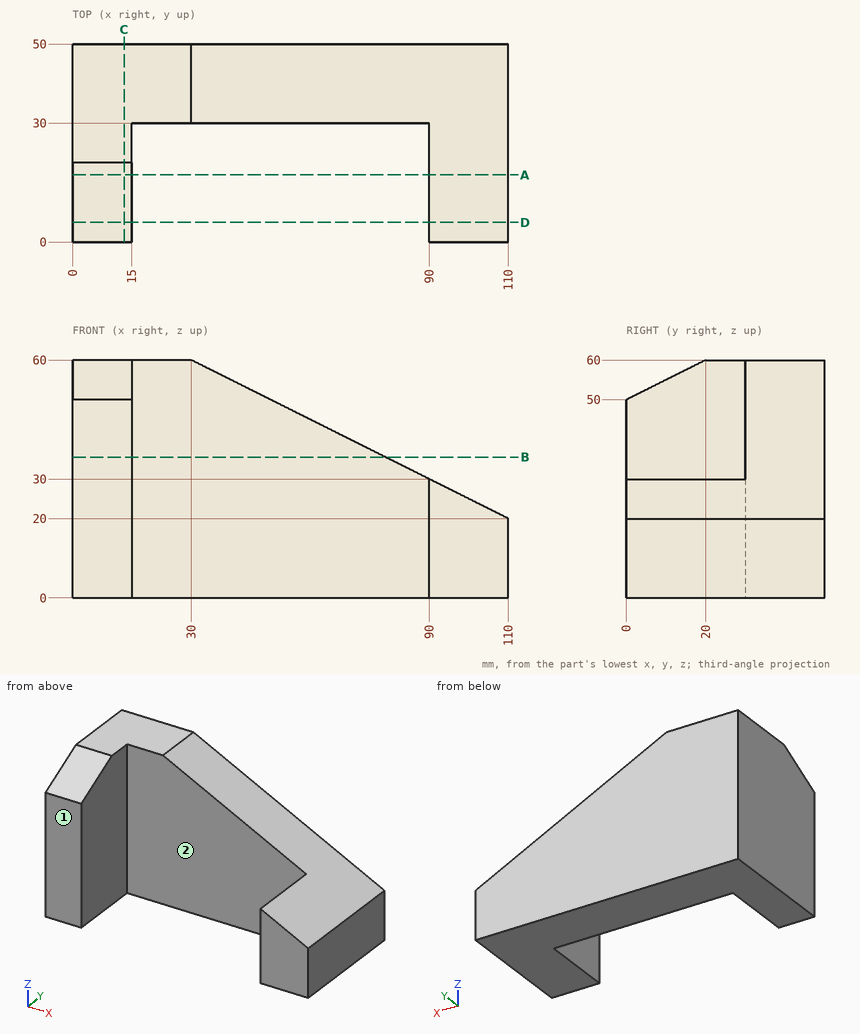
Study the drawing (mm; zero at the part's minimum x, y, z) and answer. A direction names the side the tool comes from. Round coordinates to 2 decimals unless told otherwise and drop trailing zeros. Write each loop counter-clockwise with the first axis right and the second up, starting at its lowest first coordinate (ties: lowest second). Pieces come first, ordered by that corner, then holes.
1) Which of the six approach directions +Z, -Z, +X, -X, +Y, -Y give full straight-line access (tool end or side, diameter ignored) to the marked faces 1 and 2?
2) A cutting plane is placed at A-A on y = 17. Determine the outline of the cut face in (x, z), and give its area (3 significant figures).
3) Flat-ended cylindrical pins translate along their axes: P1, Ø2, axis at x = 72.5, z = 41, coming from the -Y side; P2, Ø15, axis at y = 8.5, z = 38, coming from the +X side; P3, Ø4, axis at x = 34, y = 30.5, coming from the +Z side. Find the tip coordinate at first contact, or state that the pin passes through.
4) Consider probe 1 along X at (y, z) = (20, 19.5); probe 2 along X at (y, z) = (11, 30.5); probe 3 along Y at (x, z) = (30.5, 57). Determine where each line is inside the solid, lowest interval first.
5) A cutting plane is placed at C-C on x = 13. Determine the outline of the cut face in (y, z).
6) A cutting plane is placed at D-D on y = 5. Determine the outline of the cut face in (x, z), and give its area (3 significant figures).
7) A cutting plane is placed at B-B on z = 35.5. Determine the outline of the cut face in (x, y), and give its area (3 significant figures).
Entries:
1. face 1: +Z, -Z, +X, -X, -Y
1. face 2: +Z, -Z, -Y
2. outline: (0, 0) - (15, 0) - (15, 58.5) - (0, 58.5) - close; (90, 0) - (110, 0) - (110, 20) - (90, 30) - close
2. area: 1,380 mm2
3. P1: passes through
3. P2: stops at x = 15
3. P3: stops at z = 59
4. probe 1: x = 0 to 15, 90 to 110
4. probe 2: x = 0 to 15
4. probe 3: y = 30 to 50
5. outline: (0, 0) - (50, 0) - (50, 60) - (20, 60) - (0, 50) - close
6. outline: (0, 0) - (15, 0) - (15, 52.5) - (0, 52.5) - close; (90, 0) - (110, 0) - (110, 20) - (90, 30) - close
6. area: 1,290 mm2
7. outline: (0, 0) - (15, 0) - (15, 30) - (79, 30) - (79, 50) - (0, 50) - close
7. area: 2,030 mm2
